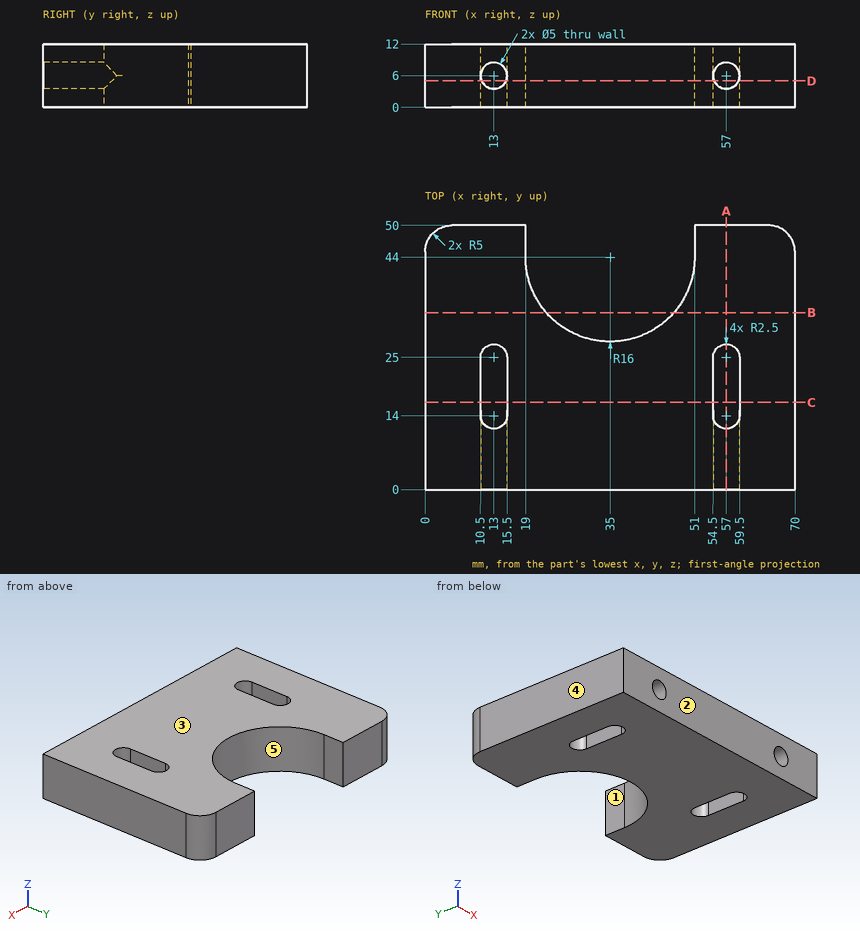
Design review of the part shown in the three views and the two pictorial views. Dimensions are in mm from the part's minimum x, y and z. A direction names the side the tool comes from. Give positions to 0.01 mm unless a question says otherwise; leave off trailing zeros. Loops run counter-clockwise (first coordinate to the right, second up) from the corner with the lowest first, then second, coordinate; pieces in that order, holes last. Notation, with made-up numbers: M -8.5,14 L 30.5,14 A8 ccw 30.5,22 Z; hole C -4,5 d7. An arc over 180 degrees is marked long. Write item = value, one per line.
Q1. We need section D-D (z = 5). Give the boundary of the cut face in (x, y).
Output values:
outline = M 0,0 L 10.71,0 L 10.71,13 A2.5 cw 10.5,14 L 10.5,25 A2.5 cw 15.5,25 L 15.5,14 A2.5 cw 15.29,13 L 15.29,0 L 54.71,0 L 54.71,13 A2.5 cw 54.5,14 L 54.5,25 A2.5 cw 59.5,25 L 59.5,14 A2.5 cw 59.29,13 L 59.29,0 L 70,0 L 70,45 A5 ccw 65,50 L 51,50 L 51,44 A16 cw 19,44 L 19,50 L 5,50 A5 ccw 0,45 Z
Q2. Draft analysis for pull direction X (two halves, no side actions). For the marked faces 3, 4 and 5, state which applies: +X half, -X half, draft (parallel to the pull), parting line (faces both ways), or undercut.
Output values:
face_3 = draft
face_4 = -X half
face_5 = undercut
Q3. For the marked faces 1 and 2, list the 3-axis set-ups (+Z, -Z, +X, -X, +Y, -Y) from which the entire face can be reached by the end or side of a thin tool; tool diameter is ignored.
Output values:
face_1 = +Z, -Z, +Y
face_2 = +Z, -Z, +X, -X, -Y
Q4. Insertion check: pin 1 (2 mm diameter, centred on x = 22, z = 8, fed in from +Y); pin 2 (3 mm diameter, centred on y = 47, z = 8, fed in from +X); pin 3 (4.5 mm diameter, centred on x = 57, z = 6, fed in from -Y); pin 4 (5 mm diameter, centred on x = 46, y = 41, fed in from -Z). Each pin has a flat end and moves straight along its axis. Give the tip position at first contact, or say it passes through.
Output values:
pin_1 = 36.25
pin_2 = 69.97
pin_3 = 26.09
pin_4 = through
Q5. We need section C-C (y = 16.5). Give the boundary of the cut face in (x, z), plus the area to 3 significant figures.
Output values:
outline = M 0,0 L 10.5,0 L 10.5,12 L 0,12 Z; M 15.5,0 L 54.5,0 L 54.5,12 L 15.5,12 Z; M 59.5,0 L 70,0 L 70,12 L 59.5,12 Z
area = 720 mm^2
Q6. We need section B-B (y = 33.5). Give the boundary of the cut face in (x, z).
Output values:
outline = M 0,0 L 22.93,0 L 22.93,12 L 0,12 Z; M 47.07,0 L 70,0 L 70,12 L 47.07,12 Z
Q7. We need section A-A (x = 57). Give the boundary of the cut face in (y, z).
Output values:
outline = M 0,0 L 11.5,0 L 11.5,3.5 L 0,3.5 Z; M 0,8.5 L 11.5,8.5 L 11.5,12 L 0,12 Z; M 27.5,0 L 50,0 L 50,12 L 27.5,12 Z
Q8. To check wall thickness, follow line 1 (X direction, y = 4.5, z = 6); line 2 (Z direction, x = 57, y = 10); line 3 (X direction, y = 27, z = 6). State the ranges of each line that lie inside material, in increasing order. Write a range as [from, to].
Output values:
line_1 = [0, 10.5], [15.5, 54.5], [59.5, 70]
line_2 = [0, 3.5], [8.5, 12]
line_3 = [0, 11.5], [14.5, 55.5], [58.5, 70]
